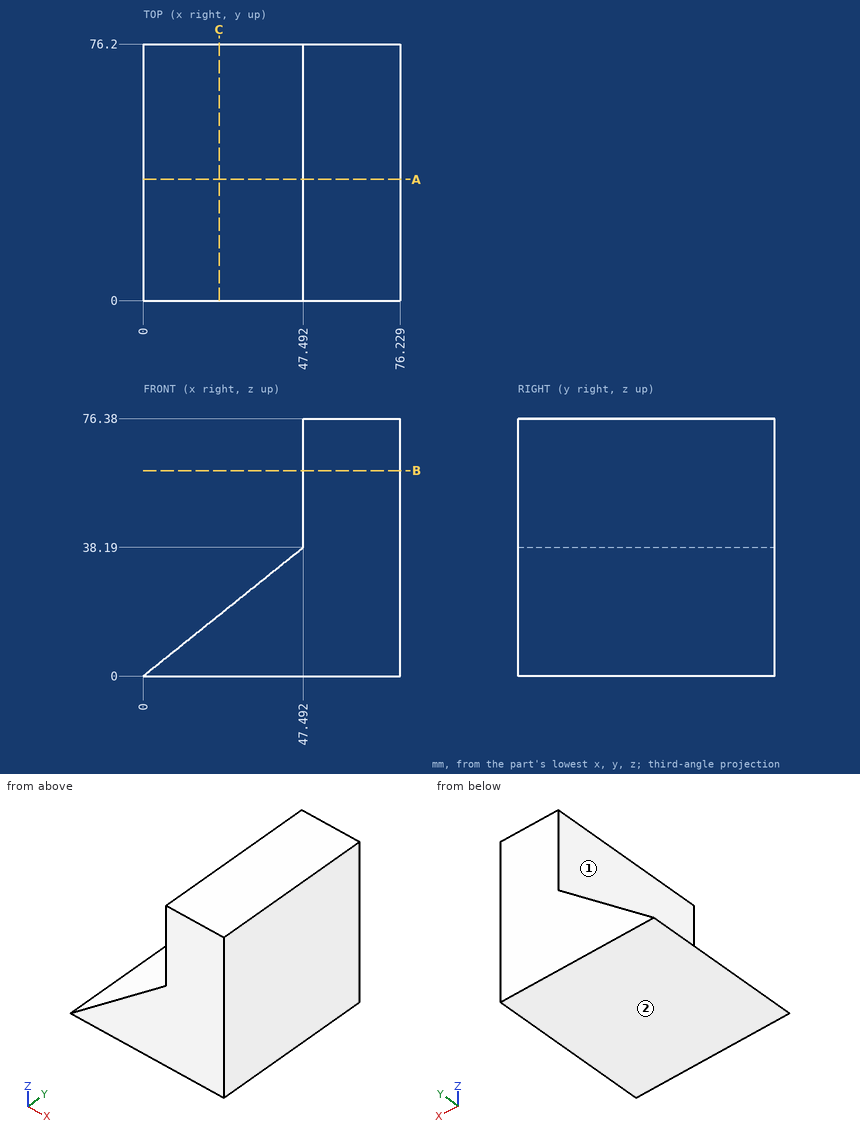
Here's the drawing with two shaded views (mm, measured from the low corner). I have some questions. A direction names the side the tool comes from. Give positions to 0.01 mm unless a question says otherwise; leave off trailing zeros. Order: outer loops, then holes, each group sorted by start corner. A loop starts at its lowest first (then second) coordinate and runs counter-clockwise, first axis right, second up. Notation, with made-up numbers: (46, 24) - (69, 24) arc R22 cw to (69, 39) - close; hole circle Ø1 at (-5.5, 73.25). An arc over 180 degrees is marked (long way). Use a Markdown table: item, result. Add a question column.
Q1. I'm going to push flat-ended pins straight in: pin 1 (10 mm diameter, centred on x = 40, y = 64.5, fed in from +Z); pin 2 (4 mm diameter, centred on x = 38, y = 18, fed in from +Z) (1 decimal). Where does each tip first touch, or does it pass through?
Q2. If we section it at A-A on y = 36: Write out the boundary of the cut face in (x, z), plus the area to 3 significant figures.
Q3. If we section it at C-C on x = 22.5: Write out the boundary of the cut face in (y, z).
Q4. Please list where these lines run through material, in increasing order: line 1 along X through (y, z) = (5, 63.5); line 2 along X through (y, z) = (70, 37); line 3 along Z through (x, y) = (9, 46).
Q5. On a 3-axis mill with a long thin cutter (end or side, diameter ignored), from which of +Z, -Z, +X, -X, +Y, -Y can I reach the whole of each face in a straight line? I mean the marked faces 1 and 2. Say none if no direction works.
Q6. If we section it at B-B on z = 61: Write out the boundary of the cut face in (x, y).
Answers follow:
| question | item | result |
|---|---|---|
| 1 | pin 1 | stops at z = 36.19 |
| 1 | pin 2 | stops at z = 32.2 |
| 2 | outline | (0, 0) - (76.23, 0) - (76.23, 76.38) - (47.49, 76.38) - (47.49, 38.19) - close |
| 2 | area | 3,100 mm^2 |
| 3 | outline | (0, 0) - (76.2, 0) - (76.2, 18.09) - (0, 18.09) - close |
| 4 | line 1 | x = 47.49 to 76.23 |
| 4 | line 2 | x = 46.01 to 76.23 |
| 4 | line 3 | z = 0 to 7.24 |
| 5 | face 1 | +Z, -X, +Y, -Y |
| 5 | face 2 | -Z, +X, -X, +Y, -Y |
| 6 | outline | (47.49, 0) - (76.23, 0) - (76.23, 76.2) - (47.49, 76.2) - close |
